Geometry: final body of the model. Coordinates: model frame, mm. A direction names the side the tool comes from. Give positions to 0.01 mm unless a question says otherwise; leave off trailing zeros. Write each loop counter-clockwise with the first axis right and the second up, starting at its lowest first coordinate (ties: lowest second). Pieces come first, ordered by that corner, then holes.
Autodesk Inventor part; units mm, degrees
ref_plane "YZ Plane" through (0, 0, 0) normal (1, 0, 0) x (0, 1, 0)
ref_plane "XZ Plane" through (0, 0, 0) normal (0, 1, 0) x (-1, 0, 0)
ref_plane "XY Plane" through (0, 0, 0) normal (0, 0, 1) x (1, 0, 0)
sketch "スケッチ1" plane through (0, 0, 0) normal (0, 1, 0) x (-1, 0, 0)
  circle A0 centre (0, 0) radius 1.15
  circle A1 centre (0, 0) radius 2
  circle A2 centre (0, 0) radius 2.9
  line L0 (-2, 0) -> (2, 0)
  line L1 (2, 0) -> (2, -2.9)
  line L2 (2, -2.9) -> (-2, -2.9)
  line L3 (-2, -2.9) -> (-2, 0)
  line L4 (0, 0) -> (0, 2.9)
  line L5 (0, 0) -> (2.9, 0)
  line L6 (2.9, 0) -> (2.9, 10)
  line L7 (2.9, 10) -> (0, 10)
  line L8 (0, 10) -> (0, 0)
  point P0 (0, 2)
  point P1 (2, -2.1)
  point P2 (-2, -2.1)
  dimension "d1" = 4
  dimension "d2" = 5.8
  dimension "d0" = 2.3
  dimension "d3" = 10
extrude "押し出し1" add sketch "スケッチ1" along normal blind 4.5 contours L5 A2 L1 | A1 L4 A2 L5 | A2 L8 L7 L6
extrude "押し出し2" add sketch "スケッチ1" along normal blind 3.5 contours A1 L3 A2 L4
extrude "押し出し3" add sketch "スケッチ1" against normal blind 1 contours L0 A1 A0 | A0 L4 A1 L0 | A0 L0 A1 L4 | L1 A2 L3 A1 | L5 A2 L1 | A1 L4 A2 L5 | A1 L3 A2 L4 | A2 L8 L7 L6
sketch "スケッチ2" plane through (-2.9, 4.5, 10) normal (0, 0, 1) x (1, 0, 0)
  line L0 (2.9, -4.5) -> (1.4, -4.5)
  line L1 (1.4, -4.5) -> (1.4, -4)
  line L2 (1.4, -4) -> (2.9, -4)
  line L3 (2.9, -4) -> (2.9, -4.5)
  dimension "d10" = 1.5
  dimension "d11" = 0.5
hole "穴1" at (-1.5, 0.5, 10) direction (0, 0, -1) diameter 1 end through all
sketch "スケッチ3" plane through (-2.9, 4.5, 10) normal (0, 0, 1) x (1, 0, 0)
  line L0 (0.9, 0) -> (0, 0)
  line L1 (0, 0) -> (4, 0)
  line L2 (4, 0) -> (4, -4)
  line L3 (4, -4) -> (0, -4)
  line L4 (0, -4) -> (0, 0)
  line L5 (0, 0) -> (3.25, 0)
  line L6 (3.25, 0) -> (3.25, -3.25)
  line L7 (3.25, -3.25) -> (0, -3.25)
  line L8 (0, -3.25) -> (0, 0)
  line L9 (0, 0) -> (1.625, 0)
  line L10 (1.625, 0) -> (1.625, -1.625)
  line L11 (1.625, -1.625) -> (0, -1.625)
  line L12 (0, -1.625) -> (0, 0)
  line L13 (0, -3.25) -> (4, -3.25)
  line L14 (4, -3.25) -> (4, 0.75)
  line L15 (4, 0.75) -> (0, 0.75)
  line L16 (0, 0.75) -> (0, -3.25)
  point P0 (2.9, -4.5)
  dimension "d19" = 4
  dimension "d20" = 4
  dimension "d21" = 3.25
  dimension "d22" = 3.25
  dimension "d33" = 4
  dimension "d34" = 4
extrude "押し出し4" add sketch "スケッチ3" along normal blind 10 and the other way blind 3 contours L1 L10 L11 L4 L0 | L0 L16 L15 L14 L1 | L1 L6 L7 L4 L11 L10 | L1 L2 L13 L6
chamfer "面取り1" distance 0.75 angle 45 1 edges at (-0.9, 5.25, 7)
chamfer "面取り2" distance 1.1 angle 45 1 edges at (1.1, 2.8752, 7)
sketch "スケッチ6" plane through (-2.9, 4.5, 20) normal (0, 0, 1) x (1, 0, 0)
  line L0 (0, 0) -> (0, 0.75)
  line L1 (0, 0.75) -> (2, 0.75)
  line L2 (2, 0.75) -> (2, -1.25)
  line L3 (2, -1.25) -> (0, -1.25)
  line L4 (0, -1.25) -> (0, 0.75)
  circle A0 centre (2, -1.25) radius 1.075
  point P0 (2.9, -4.5)
  dimension "d41" = 2
  dimension "d42" = 2
  dimension "d43" = 2.15
extrude "押し出し6" cut sketch "スケッチ6" against normal blind 10 contours A0 L2 L3 | L3 L2 A0
properties part number "srod1.7right"
Q1. Section C-C on x = -2.45. Output: boundary loops of the cut face in (y, z).
Filled sheet:
outline: (-1, -1.55) - (4.5, -1.55) - (4.5, 7) - (5.25, 7.75) - (5.25, 20) - (1.25, 20) - (1.25, 10) - (-1, 10) - close
Q2. Pull-direction query (X, two-part tool) for faces 6 (the cylindrical face through (0.91, -0.49, -0.7)), 7 (the flat face through (-1, 0, 10)), 8 (the flat face through (1.1, 3, 14)); classes: released by +X, released by -X, zero draft, split by the parting line, or undercut.
Filled sheet:
face 6: undercut
face 7: zero draft
face 8: released by +X
Q3. Access query for faces 1 (the flat face through (0, 0, -2)), 2 (the flat face through (-2, 2, 20)), 3 (the cylindrical face through (-1.04, 4.316, 15.07)), 4 (the flat face through (0.6, 3.2, 7.6)), 5 (the flat face through (2, 3.5, 1)). Directions: +Z, -Z, +X, -X, +Y, -Y. A direction counts if a zero-diameter tool reaches every point of the face in a straight line with its end or side. Return the directions, or none.
Filled sheet:
face 1: -Z, +Y
face 2: +Z, +X, -X, +Y, -Y
face 3: +Z
face 4: +X, +Y, -Y
face 5: -Z, +X, +Y
Q4. Pin query (flat end, axial travel): P1, Ø1.2, axis at y = 3, z = 12, coming from the +X side; P2, Ø0.6, axis at x = -1, y = 3, coming from the +Z side; P3, Ø1, axis at y = 1.5, z = -1.5, coming from the +X side; P4, Ø3, axis at x = -1, y = 4, coming from the +Z side. Return the tip coordinate at first contact, or that it passes through.
Filled sheet:
P1: stops at x = 1.1
P2: stops at z = 10
P3: stops at x = 2.72
P4: stops at z = 20
Q5. Ray query, line 1 along X through (y, z) = (0.5, 3); line 2 along X through (y, z) = (3.25, 15.5) (3 decimals); line 3 along Y through (x, z) = (-1.45, 2). Return the intervals inside material, ascending.
Filled sheet:
line 1: x = -2.9 to -2, -1 to 0
line 2: x = -2.9 to -1.975, 0.175 to 1.1
line 3: y = -1 to 0, 1 to 4.5
Q6. Section D-D on z = 17.5. Output: boundary loops of the cut face in (x, y) (3 decimals), plus the area to 3 significant figures.
Filled sheet:
outline: (-2.9, 1.25) - (1.1, 1.25) - (1.1, 5.25) - (-2.9, 5.25) - close; hole circle Ø2.15 at (-0.9, 3.25)
area: 12.4 mm2
Q7. Section A-A on z = 6.75. Output: boundary loops of the cut face in (x, y), plus the area to 3 significant figures.
Filled sheet:
outline: (-2.9, -1) - (0, -1) - (0, 4.5) - (-2.9, 4.5) - close; hole circle Ø1 at (-1.5, 0.5)
area: 15.2 mm2
